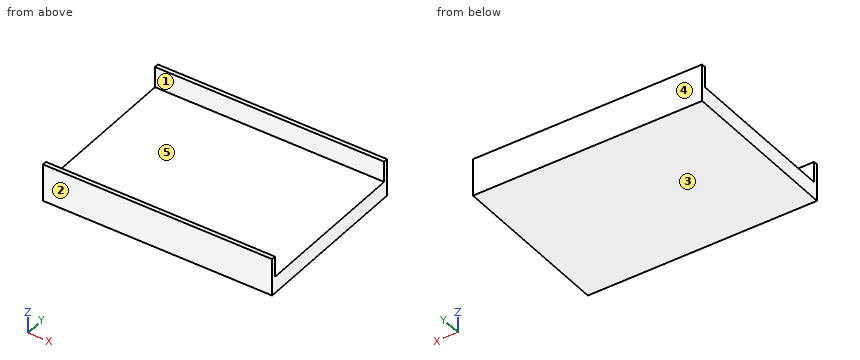
from build123d import *

# Parameters (mm, degrees)
F0_W     = 55
F0_H     = 40
F1_DEPTH = 4
F2_W     = 55
F2_H     = 1
F3_DEPTH = 5
F4_W     = 55
F4_H     = 1
F5_DEPTH = 5


# Not quite as in the source:
# - the program builds the solid bodies; features that only make, move or delete a surface that nothing else refers to are left out


with BuildPart() as f1:
    # F0 (on Top) → F1 (new body)
    with BuildSketch(Plane.XY):
        Rectangle(F0_W, F0_H)
    extrude(amount=F1_DEPTH)

    # F2 (on face) → F3 (join)
    with BuildSketch(Plane.XY.offset(4)):
        with Locations((0, -19.5)):
            Rectangle(F2_W, F2_H)
    extrude(amount=F3_DEPTH)

    # F4 (on face) → F5 (join)
    with BuildSketch(Plane.XY.offset(4)):
        with Locations((0, 19.5)):
            Rectangle(F4_W, F4_H)
    extrude(amount=F5_DEPTH)


solid = f1.part
Build history of the part. All positions in model axes, mm. Face numbers are marked on the shaded views. A direction names the side the tool comes from. Round coordinates to 2 decimals unless told otherwise and drop trailing zeros. Order: outer loops, then holes, each group sorted by start corner. A loop starts at its lowest first (then second) coordinate and runs counter-clockwise, first axis right, second up. Notation, with made-up numbers: M -14.75,45.25 L 35.25,45.25 A33 ccw 35.25,81.25 Z; hole C 1,41.25 d5. An arc over 180 degrees is marked long. Use CSV: the item, a comma, the result in double quotes. Start each with the question number.
(1) Cut at B-B on x = -1. List the corners of the cut face in (y, z), then the cut area to 3 significant figures.
(2) Cut at C-C on y = -1. List the corners of the cut face in (x, z).
(3) Mould opens along Y. For the marked faces 1, 2 and 3 say: +Y half, -Y half, draft (parallel to the pull), parting line (faces both ways), or undercut.
(4) Tool access for the marked faces 4 and 5: list every direction of +Z, -Z, +X, -X, +Y, -Y with a clear straight run to the whole face (end or side of a thin tool).
(5) Drill centre lines: probe 1 along Y at (x, z) = (-7.5, 8.5); probe 2 along Z at (x, y) = (17.5, -18). Where is each one in solid material? Low to high.
(6) Flat gauge pins, fed straight in: P1, Ø12, axis at x = 17.5, y = -2.5, coming from the +Z side; P2, Ø12, axis at x = 14, y = 2, coming from the -Z side. Where does each tip first touch, or does it go through?
(7) Cut at A-A on z = 7.75. List the corners of the cut face in (x, y), then the cut area to 3 significant figures.
Findings:
1,outline,"M -20,0 L 20,0 L 20,9 L 19,9 L 19,4 L -19,4 L -19,9 L -20,9 Z"
1,area,"170 mm^2"
2,outline,"M -27.5,0 L 27.5,0 L 27.5,4 L -27.5,4 Z"
3,face 1,"undercut"
3,face 2,"-Y half"
3,face 3,"draft"
4,face 4,"+Z, -Z, +X, -X, +Y"
4,face 5,"+Z, +X, -X"
5,probe 1,"y = -20 to -19, 19 to 20"
5,probe 2,"z = 0 to 4"
6,P1,"stops at z = 4"
6,P2,"stops at z = 0"
7,outline,"M -27.5,-20 L 27.5,-20 L 27.5,-19 L -27.5,-19 Z; M -27.5,19 L 27.5,19 L 27.5,20 L -27.5,20 Z"
7,area,"110 mm^2"
